Geometry: see drawing. Coordinates: mm, zero at the bounding-box minimum. Give positions to 0.01 mm unless a question says otherwise; leave off trailing zeros. Write each loop counter-clockwise with the first axis right and the second up, starting at its lowest first coordinate (ties: lowest second). Pieces come first, ordered by that corner, then holes. Notation, with made-up numbers: (61.25, 7) - (118.25, 7) arc R18 cw to (118.25, 33) - close; hole circle Ø9 at (25, 64). An arc over 180 degrees is marked (long way). Return JSON: item names as keys, results as strings.
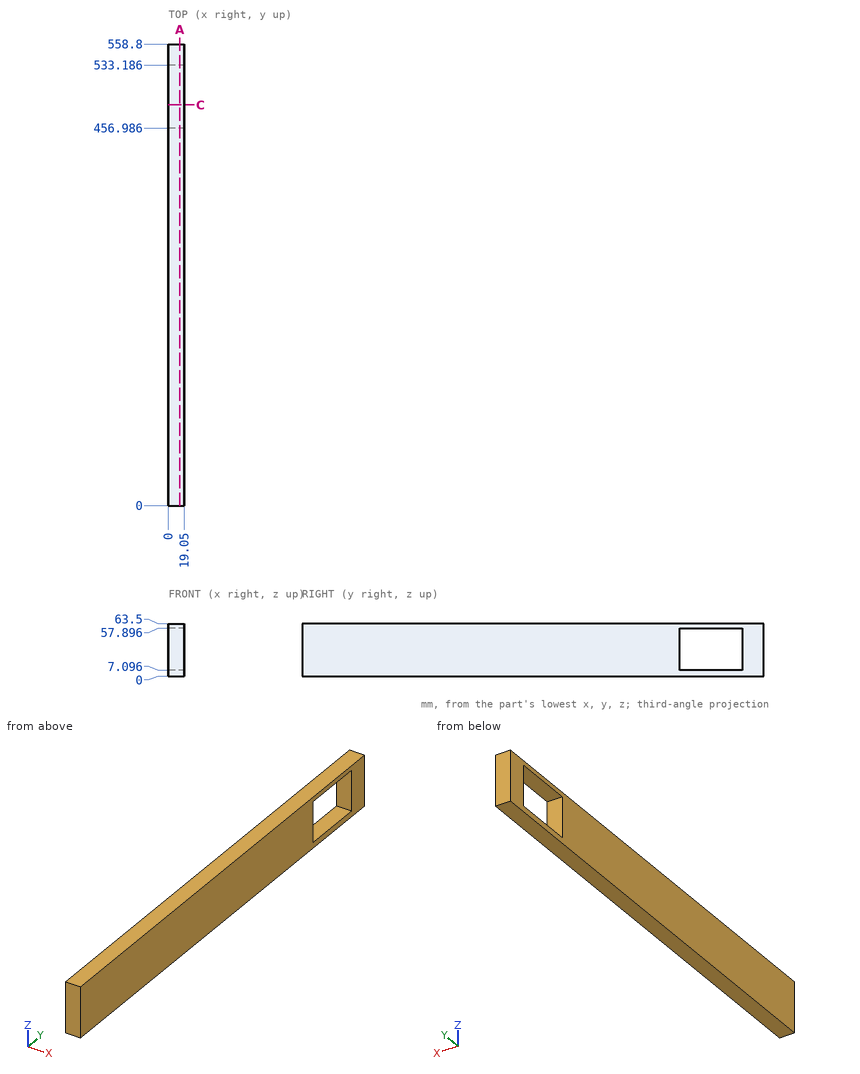
Q1. Section query C-C, the plane y = 485. Return the cut outline in (x, z).
Answer key:
{"outline": "(0, 0) - (19.05, 0) - (19.05, 7.1) - (0, 7.1) - close; (0, 57.9) - (19.05, 57.9) - (19.05, 63.5) - (0, 63.5) - close"}
Q2. Pin query (flat end, axial travel): P1, Ø5, axis at x = 2.5, y = 63, coming from the -Z side. Return the tip coordinate at first contact, or that it passes through.
Answer key:
{"P1": "stops at z = 0"}
Q3. Section query A-A, the plane x = 14. Return the cut outline in (y, z) (1 decimal), plus the area to 3 significant figures.
Answer key:
{"outline": "(0, 0) - (558.8, 0) - (558.8, 63.5) - (0, 63.5) - close; hole (457, 7.1) - (533.2, 7.1) - (533.2, 57.9) - (457, 57.9) - close", "area": "31,600 mm^2"}
Q4. Material intervals for probe 1 along Y at (x, z) = (10.25, 17) (1 decimal); probe 2 along Z at (x, y) = (15.5, 497), sorted ascending. Write a range as [from, to].
Answer key:
{"probe 1": "y = [0, 457], [533.2, 558.8]", "probe 2": "z = [0, 7.1], [57.9, 63.5]"}
